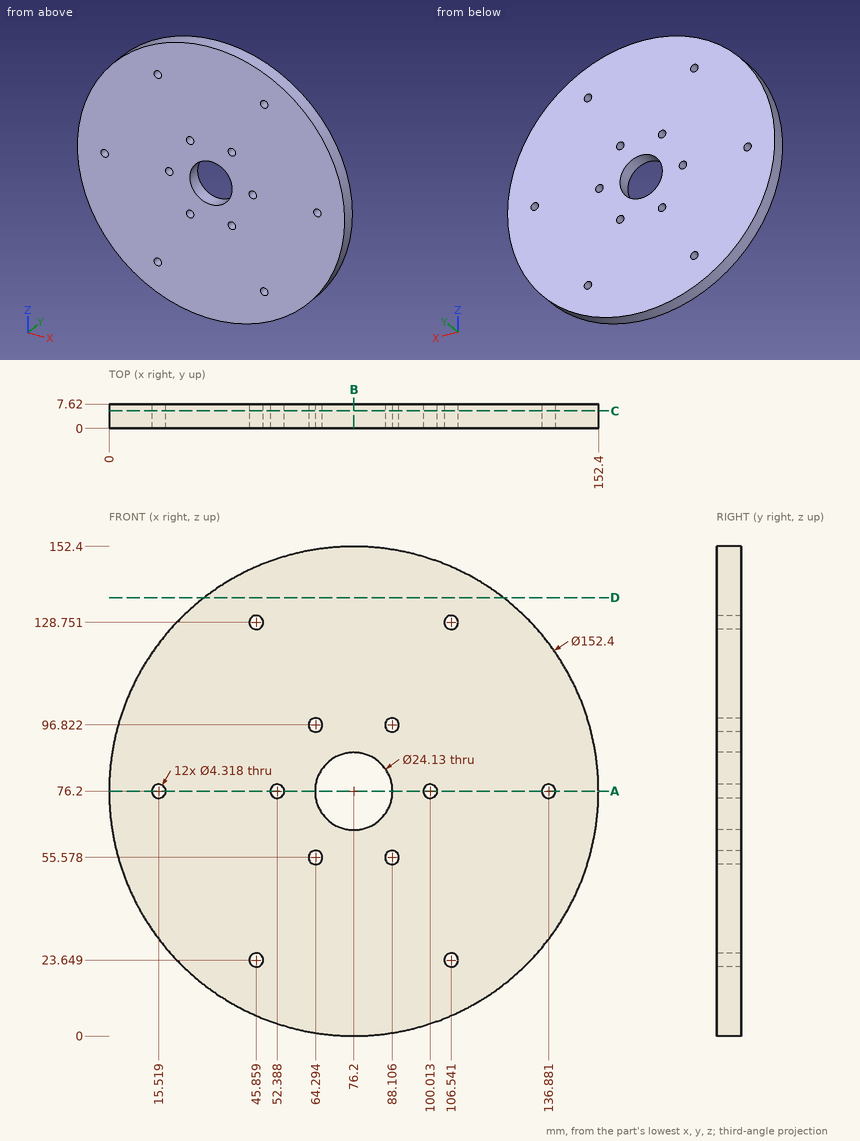
Job drawing, mm, ordinate dimensions from the low corner. One solid piece. Coordinates: 2 decimals unless noted, no trailing zeros. Loops run counter-clockwise (first coordinate to the right, second up) from the corner with the lowest first, then second, coordinate; pieces in that order, holes last. Notation, with made-up numbers: (69, -36.75) - (123, -36.75) arc R28 cw to (123, -16.75) - close; hole circle Ø2 at (68.5, 57.5). An arc over 180 degrees is marked (long way). Answer as a JSON object with one key per item and string values. Group by question number.
(1) Cut at D-D (z = 136.5). Give the cut face in (x, y).
(2) Flat gauge pins, fed straight in: pin 1 (5.5 mm diameter, centred on x = 45.86, z = 128.75, fed in from +Y); pin 2 (3 mm diameter, centred on x = 106, y = 2, fed in from +Z); pin 3 (2 mm diameter, centred on x = 117.5, y = 5.5, fed in from -Z); pin 4 (3 mm diameter, centred on y = 1, z = 21.5, fed in from +X) (1 decimal). Where does each tip first touch, or does it go through?
(3) Cut at C-C (y = 5.5). State how many separate pieces and enclosed holes the cut face has, then the cut area to 3 significant figures.
(4) Probe line 1 along Z through (x, y) = (77, 2.25) (1 decimal); line 2 along X through (y, z) = (0.5, 77) (1 decimal); line 3 along X through (y, z) = (3.5, 22.5) (1 decimal). List the from-to ranges inside material, lowest first.
(5) Cut at A-A (z = 76.2). Give the cut face in (x, y) (1 decimal).
(6) Cut at B-B (x = 76.2). Give the cut face in (y, z) (1 decimal).
Geometry says:
{
 "1": {"outline": "(29.61, 0) - (122.79, 0) - (122.79, 7.62) - (29.61, 7.62) - close"},
 "2": {"pin 1": "stops at y = 7.62", "pin 2": "stops at z = 146.95", "pin 3": "stops at z = 11.53", "pin 4": "stops at x = 130.8"},
 "3": {"separate pieces": "1", "enclosed holes": "13", "area": "17,600 mm^2"},
 "4": {"line 1": "z = 0 to 64.2, 88.2 to 152.4", "line 2": "x = 0 to 13.5, 17.5 to 50.4, 54.4 to 64.2, 88.2 to 98, 102 to 134.9, 138.9 to 152.4", "line 3": "x = 22.1 to 44, 47.7 to 104.7, 108.4 to 130.3"},
 "5": {"outline": "(0, 0) - (13.4, 0) - (13.4, 7.6) - (0, 7.6) - close; (17.7, 0) - (50.2, 0) - (50.2, 7.6) - (17.7, 7.6) - close; (54.5, 0) - (64.1, 0) - (64.1, 7.6) - (54.5, 7.6) - close; (88.3, 0) - (97.9, 0) - (97.9, 7.6) - (88.3, 7.6) - close; (102.2, 0) - (134.7, 0) - (134.7, 7.6) - (102.2, 7.6) - close; (139, 0) - (152.4, 0) - (152.4, 7.6) - (139, 7.6) - close"},
 "6": {"outline": "(0, 0) - (7.6, 0) - (7.6, 64.1) - (0, 64.1) - close; (0, 88.3) - (7.6, 88.3) - (7.6, 152.4) - (0, 152.4) - close"}
}
